Source: CAD feature listing. Evaluate the final solid. Frame: model axes, mm. Face numbers are marked on the shaded views. A direction names the side the tool comes from. Round coordinates to 2 decimals unless told otherwise and drop trailing zeros. Loops run counter-clockwise (first coordinate to the right, second up) from the corner with the lowest first, then second, coordinate; pieces in that order, holes last. Notation, with made-up numbers: M 20,69 L 76,69 A27 ccw 76,90 Z; hole C 31,-27.75 d2. An arc over 180 degrees is marked long. Answer as a JSON object with one key per item and string values.
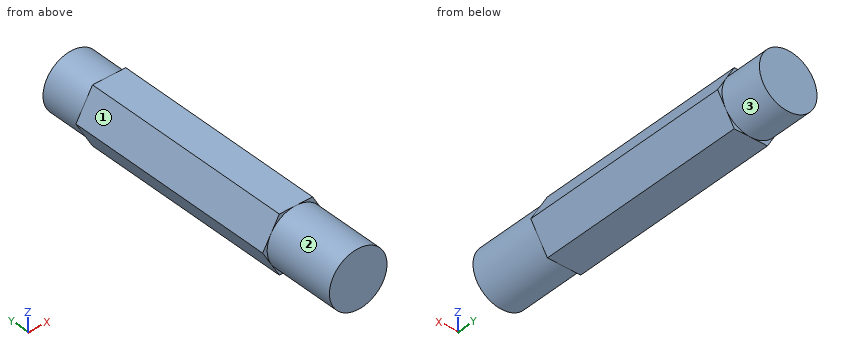
from build123d import *

# Parameters (mm, degrees)
BOSS_EXTRUDE1_DEPTH = 7.5
SKETCH2_R           = 2
BOSS_EXTRUDE3_DEPTH = 3
BOSS_EXTRUDE4_START = 5
SKETCH4_R           = 2
BOSS_EXTRUDE4_DEPTH = 5


with BuildPart() as part:
    # Sketch1 → Boss-Extrude1 (new, symmetric)
    with BuildSketch(Plane(origin=(0, 0, 0), x_dir=(1, 0, 0), z_dir=(0, 1, 0))):
        Polygon((-2.309401077, 0), (-1.154700538, -2), (1.154700538, -2), (2.309401077, 0), (1.154700538, 2), (-1.154700538, 2), align=None)
    extrude(amount=BOSS_EXTRUDE1_DEPTH, both=True)

    # Sketch2 → Boss-Extrude3 (add)
    with BuildSketch(Plane(origin=(0, 7.5, 0), x_dir=(1, 0, 0), z_dir=(0, 1, 0))):
        with Locations(Location((0, 0, 0), (0, 0, 270))):
            Circle(SKETCH2_R)
    extrude(amount=BOSS_EXTRUDE3_DEPTH)

    # Sketch4 → Boss-Extrude4 (add)
    with BuildSketch(Plane.XZ.offset(7.5).offset(BOSS_EXTRUDE4_START)):
        with Locations(Location((0, 0, 0), (0, 0, 90))):
            Circle(SKETCH4_R)
    extrude(amount=-BOSS_EXTRUDE4_DEPTH)


solid = part.part
Item 1: Contact query for flat-ended pins moving along their axis: pin 1 Ø0.6 at (x, z) = (-2, -0.5) entering from -Y; pin 2 Ø1.5 at (y, z) = (-6.5, -1) entering from -X; pin 3 Ø2 at (y, z) = (-3.5, -1.5) entering from +X. Output: stop coordinate, or through.
Answer sheet:
{"pin 1": "stops at y = -12.5", "pin 2": "stops at x = -2.17", "pin 3": "stops at x = 2.02"}
Item 2: Section A-A on z = 0.5. Return the cut outline in (x, y).
Answer sheet:
{"outline": "M -2.02,-7.5 L -1.94,-7.5 L -1.94,-12.5 L 1.94,-12.5 L 1.94,-7.5 L 2.02,-7.5 L 2.02,7.5 L 1.94,7.5 L 1.94,10.5 L -1.94,10.5 L -1.94,7.5 L -2.02,7.5 Z"}
Item 3: Section B-B on y = 4.75. Return the cut outline in (x, z), then the cut area to 3 significant figures.
Answer sheet:
{"outline": "M -2.31,0 L -1.15,-2 L 1.15,-2 L 2.31,0 L 1.15,2 L -1.15,2 Z", "area": "13.9 mm²"}
Item 4: Section C-C on x = -1.4. Return the cut outline in (y, z).
Answer sheet:
{"outline": "M -12.5,-1.43 L -7.5,-1.43 L -7.5,-1.58 L 7.5,-1.58 L 7.5,-1.43 L 10.5,-1.43 L 10.5,1.43 L 7.5,1.43 L 7.5,1.58 L -7.5,1.58 L -7.5,1.43 L -12.5,1.43 Z"}
Item 5: Line query: probe 1 along X at (y, z) = (8.75, 0.1); probe 2 along Z at (x, y) = (1.7, 8.75). Output: solid intervals per line, ascending. Write a range as from..to.
Answer sheet:
{"probe 1": "x = -2..2", "probe 2": "z = -1.05..1.05"}
Item 6: Access query for the marked faces 1, 2 and 3. Directions: +Z, -Z, +X, -X, +Y, -Y. A direction counts if a zero-diameter tool reaches every point of the face in a straight line with its end or side. Return the directions, or none.
Answer sheet:
{"face 1": "+Z, -X, +Y, -Y", "face 2": "-Y", "face 3": "+Y"}
